Design review of the part built by this model. Coordinates are the model's own, in mm. A direction names the side the tool comes from. Give positions to 0.01 mm unless a question says otherwise; leave off trailing zeros. Loops run counter-clockwise (first coordinate to the right, second up) from the corner with the lowest first, then second, coordinate; pieces in that order, holes last.
from build123d import *

# Parameters (mm, degrees)
F0_W     = 177.8
F0_H     = 127
F1_DEPTH = 76.2
F2_W     = 76.2
F2_H     = 92.075
F3_DEPTH = 82.55
F4_W     = 76.2
F4_H     = 6.35
F5_DEPTH = 88.9


with BuildPart() as f1:
    # F0 (on Front) → F1 (new body)
    with BuildSketch(Plane.XZ):
        with Locations((88.9, 63.5)):
            Rectangle(F0_W, F0_H)
    extrude(amount=F1_DEPTH)

    # F2 (on face) → F3 (cut)
    with BuildSketch(Plane.YZ.offset(177.8)):
        with Locations((-38.1, 80.9625)):
            Rectangle(F2_W, F2_H)
    extrude(amount=-F3_DEPTH, mode=Mode.SUBTRACT)

    # F4 (on face) → F5 (cut)
    with BuildSketch(Plane.YZ.offset(177.8)):
        with Locations((-38.1, 31.75)):
            Rectangle(F4_W, F4_H)
    extrude(amount=-F5_DEPTH, mode=Mode.SUBTRACT)


solid = f1.part
Q1. Take a section at B-B (z = 37.5). Give the boundary of the cut face in (x, y).
Results:
outline: (0, -76.2) - (95.25, -76.2) - (95.25, 0) - (0, 0) - close
Q2. Take a section at A-A (y = -38.5). Give the boundary of the cut face in (x, z) (3 decimals).
Results:
outline: (0, 0) - (177.8, 0) - (177.8, 28.575) - (88.9, 28.575) - (88.9, 34.925) - (95.25, 34.925) - (95.25, 127) - (0, 127) - close
Q3. Draft analysis for pull direction Z (two halves, no side actions). For faces 1 (the face through (0, -38, 63)), 2 (the face through (88.9, -39, 32)), 3 (the face through (47, -38, 127)), state which applies: pulls with the +Z half, pulls with the -Z half, needs draft (parallel to the pull), parting line crosses it, or undercut.
Results:
face 1: needs draft
face 2: undercut
face 3: pulls with the +Z half
Q4. Insertion check: pin 1 (12 mm diameter, centred on y = -13, z = 110, fed in from +X); pin 2 (1.9 mm diameter, centred on y = -29.5, z = 32.5, fed in from +X). Each pin has a flat end and moves straight along its axis. Give the tip position at first contact, or say it passes through.
Results:
pin 1: stops at x = 95.25
pin 2: stops at x = 88.9
Q5. Take a section at C-C (x = 120). Give the boundary of the cut face in (y, z) (3 decimals).
Results:
outline: (-76.2, 0) - (0, 0) - (0, 28.575) - (-76.2, 28.575) - close
Q6. Tool access review of faces 4 (the face through (95.25, -39, 82)), 5 (the face through (177.8, -38, 14)), 6 (the face through (92, -39, 34.925)): name each direction out of +Z, -Z, +X, -X, +Y, -Y from which nothing blocks a thin tool from reaching the whole face with its end or side.
Results:
face 4: +Z, +X, +Y, -Y
face 5: +Z, -Z, +X, +Y, -Y
face 6: +X, +Y, -Y
Q7. Wall thickness on line 1 (Z direction, x = 105.5, y = -14.5) (3 decimals); line 2 (X direction, y = -65, z = 121.5): over which ranges is each line inside the solid? List them lowest first.
Results:
line 1: z = 0 to 28.575
line 2: x = 0 to 95.25
